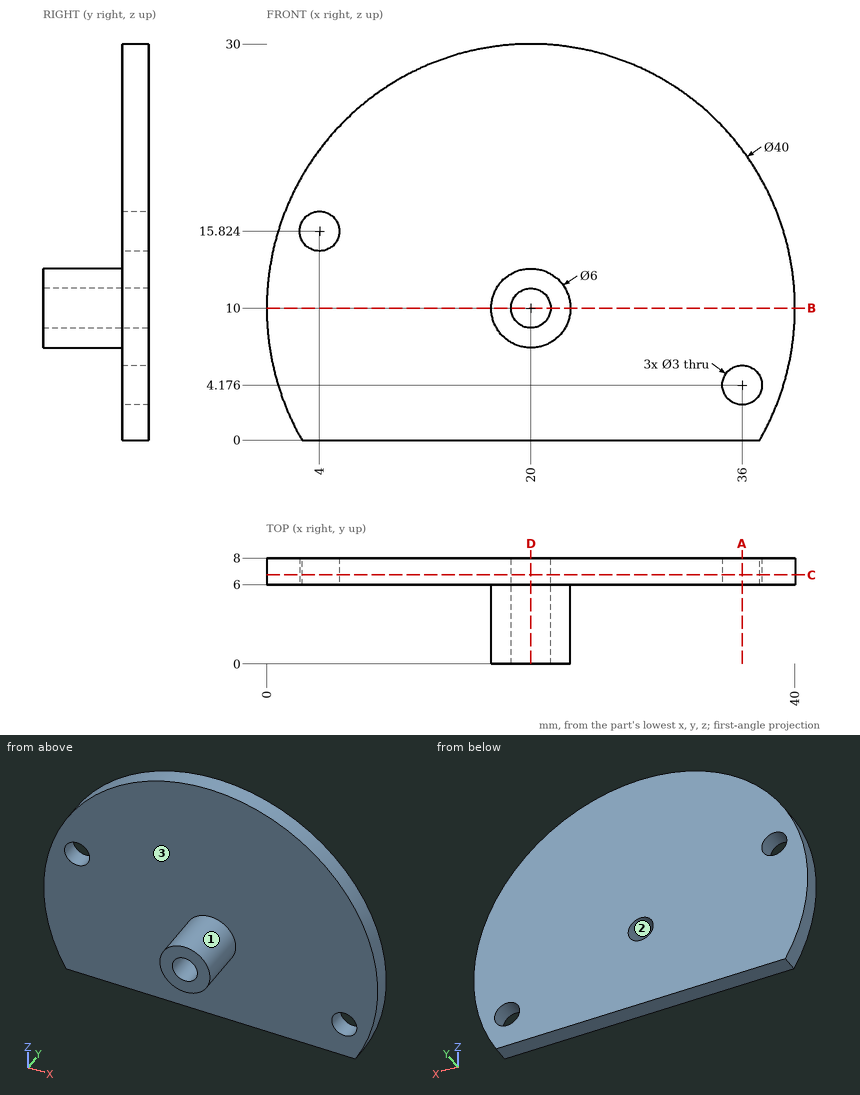
The drawing under review shows one solid part. Ordinate dimensions are in mm from its lowest x, y, z. Give positions to 0.01 mm unless a question says otherwise; leave off trailing zeros. Write each loop counter-clockwise with the first axis right and the second up, starting at its lowest first coordinate (ties: lowest second). Pieces come first, ordered by that corner, then holes.
1. Draft analysis for pull direction Z (two halves, no side actions). For the marked faces 1, 2 and 3, state which applies: +Z half, -Z half, draft (parallel to the pull), parting line (faces both ways), or undercut.
2. Add section C-C, the plane y = 6.75. Write out the cut boundary in (x, z).
3. Add section B-B, the plane z = 10. Write out the cut boundary in (x, y).
4. Wall thickness on L1, parallel to X at y = 4.25, z = 10; L2, parallel to X at y = 6.25, z = 10; L3, parallel to Y at x = 34, z = 20.75: over which ranges is each line inside the solid? List them lowest first.
5. Add section A-A, the plane x = 36. Write out the cut boundary in (y, z).
6. Add section D-D, the plane x = 20. Write out the cut boundary in (y, z).
7. For P1, Ø2, axis at x = 19, z = 18.5, coming from the -Y side, flat-tipped, find the tip position at first contact; note if it passes through.
Worked answers:
1. face 1: parting line
1. face 2: undercut
1. face 3: draft
2. outline: (2.68, 0) - (37.32, 0) arc R20 ccw (long way) to start; hole circle Ø3 at (4, 15.82); hole circle Ø3 at (20, 10); hole circle Ø3 at (36, 4.18)
3. outline: (0, 6) - (17, 6) - (17, 0) - (18.5, 0) - (18.5, 8) - (0, 8) - close; (21.5, 0) - (23, 0) - (23, 6) - (40, 6) - (40, 8) - (21.5, 8) - close
4. L1: x = 17 to 18.5, 21.5 to 23
4. L2: x = 0 to 18.5, 21.5 to 40
4. L3: y = 6 to 8
5. outline: (6, 0) - (8, 0) - (8, 2.68) - (6, 2.68) - close; (6, 5.68) - (8, 5.68) - (8, 22) - (6, 22) - close
6. outline: (0, 7) - (6, 7) - (6, 0) - (8, 0) - (8, 8.5) - (0, 8.5) - close; (0, 11.5) - (8, 11.5) - (8, 30) - (6, 30) - (6, 13) - (0, 13) - close
7. P1: stops at y = 6
